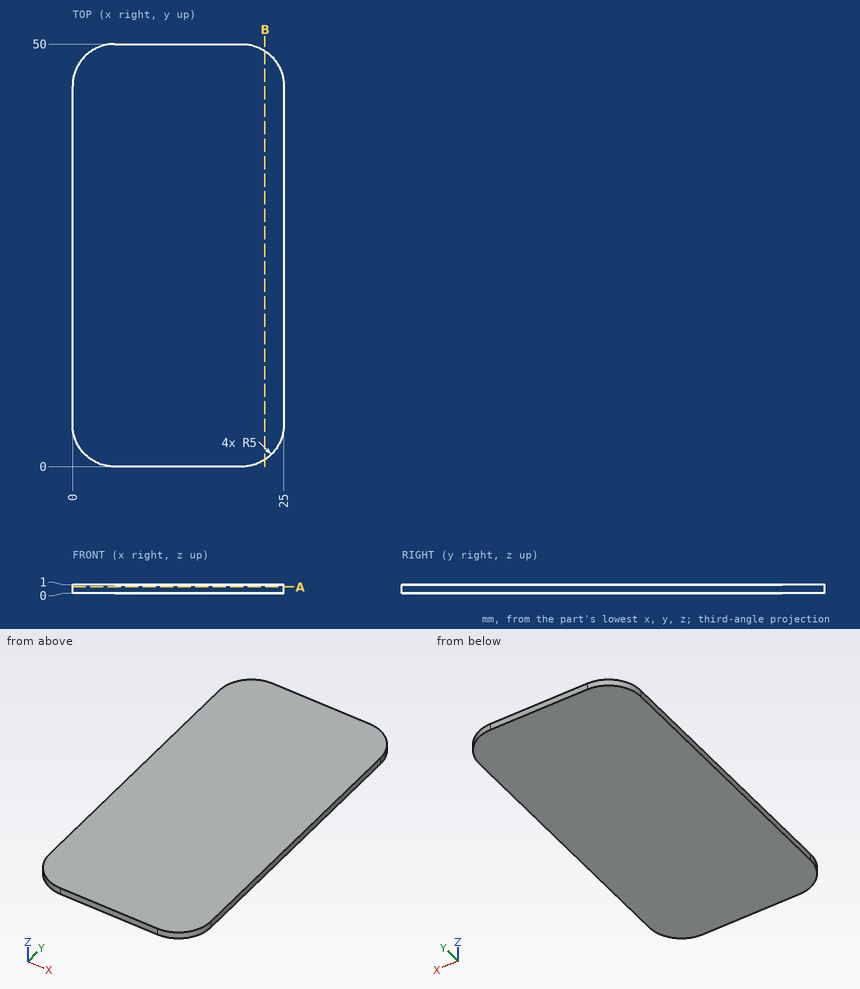
Input: dimensioned drawing with shaded views. Units: mm. Origin: part minimum x, y, z. Give positions to 0.01 mm unless a question says otherwise; leave off trailing zeros. Write each loop counter-clockwise with the first axis right and the second up, starting at its lowest first coordinate (ties: lowest second). Pieces come first, ordered by that corner, then holes. Notation, with made-up numbers: M 64.5,-37 L 85.5,-37 A9 ccw 85.5,-29 Z; hole C 35.25,15 d5. An arc over 180 degrees is marked long. Return JSON: item names as keys, results as strings. Group by question number.
1) Material intervals for line 1 along X through (y, z) = (2, 0.55); line 2 along Y through (x, z) = (20.75, 0.15); line 3 along X through (y, z) = (47, 0.55), sorted ascending. Write a range as [from, to].
2) Cut plane B-B, the plane x = 22.75. Output: boundary loops of the cut face in (y, z).
3) Cut plane A-A, the plane z = 0.75. Output: boundary loops of the cut face in (x, y).
Recorded:
{
 "1": {"line 1": "x = [1, 24]", "line 2": "y = [0.06, 49.94]", "line 3": "x = [0.42, 24.58]"},
 "2": {"outline": "M 0.82,0 L 49.18,0 L 49.18,1 L 0.82,1 Z"},
 "3": {"outline": "M 0,5 A5 ccw 5,0 L 20,0 A5 ccw 25,5 L 25,45 A5 ccw 20,50 L 5,50 A5 ccw 0,45 Z"}
}
